Can you work these out from the model? Positions are in its coordinate system, mm. Face numbers are marked on the shaded views. Give positions to 0.01 mm unless a question says otherwise; leave off trailing zeros. Loops run counter-clockwise (first coordinate to the right, second up) from the corner with the lowest first, then second, coordinate; pieces in that order, holes last. Notation, with made-up numbers: M 69,10.5 L 100,10.5 A33 cw 100,42.5 Z; hole C 73,-23 d1. An arc over 180 degrees is marked long. One line per item, written item: value. Start each with the question number.
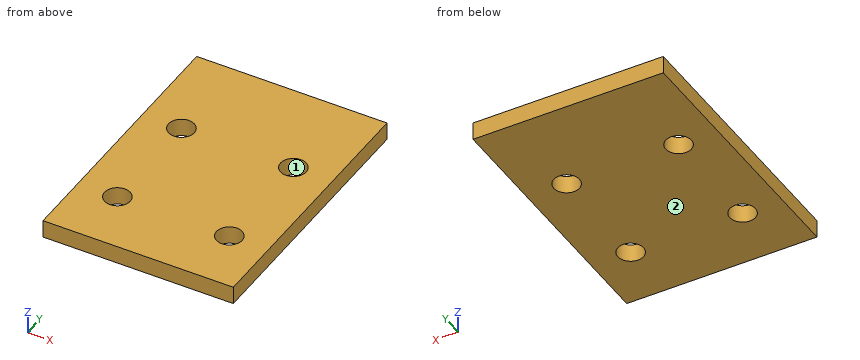
from build123d import *

# Parameters (mm, degrees)
SKETCH_1_W             = 170
SKETCH_1_H             = 240
SKETCH_1_R             = 11.5
SM_BASE_FLANGE_1_DEPTH = 16


# Sheet-metal steps are written as plain solids
with BuildPart() as part:
    # Sketch 1 → Базовая кромка1 (new body)
    with BuildSketch(Plane.XY):
        with Locations((85, -120)):
            Rectangle(SKETCH_1_W, SKETCH_1_H)
        with Locations((135, -185)):
            Circle(SKETCH_1_R, mode=Mode.SUBTRACT)
        with Locations((135, -85)):
            Circle(SKETCH_1_R, mode=Mode.SUBTRACT)
        with Locations(Location((35, -85, 0), (0, 0, 180))):
            Circle(SKETCH_1_R, mode=Mode.SUBTRACT)
        with Locations(Location((35, -185, 0), (0, 0, 180))):
            Circle(SKETCH_1_R, mode=Mode.SUBTRACT)
    extrude(amount=-SM_BASE_FLANGE_1_DEPTH)


solid = part.part
Q1. If we mould it in two halves opening along X, with no side actions, what happens to the marked faces 1 and 2? For each: released by +X, released by -X, zero draft, split by the parting line, or undercut.
Q2. For P1, Ø3, axis at x = 123.5, y = -139, coming from the +Z side, with a flat end and sliding along its axis, tell me the tip position at first contact or that it passes through.
Q3. If we section it at A-A, the plane y = -185: Write out the boundary of the cut face in (x, z), plus the area to 3 significant figures.
Q4. I need wall thicknesses on line 1 along Y through (x, z) = (135, -7); line 2 along Y through (x, z) = (42, -9.25); line 3 along X through (y, z) = (-88, -2.25). Which ranges of each line are inside material? Lowest first, please.
Q5. If we section it at C-C, the plane x = 141: Write out the boundary of the cut face in (y, z).
Q6. If we section it at B-B, the plane z = -13.5: Write out the boundary of the cut face in (x, y).
Response:
1. face 1: undercut
1. face 2: zero draft
2. P1: z = 0
3. outline: M 0,-16 L 23.5,-16 L 23.5,0 L 0,0 Z; M 46.5,-16 L 123.5,-16 L 123.5,0 L 46.5,0 Z; M 146.5,-16 L 170,-16 L 170,0 L 146.5,0 Z
3. area: 1,980 mm^2
4. line 1: -240 to -196.5, -173.5 to -96.5, -73.5 to 0
4. line 2: -240 to -194.12, -175.88 to -94.12, -75.88 to 0
4. line 3: 0 to 23.9, 46.1 to 123.9, 146.1 to 170
5. outline: M -240,-16 L -194.81,-16 L -194.81,0 L -240,0 Z; M -175.19,-16 L -94.81,-16 L -94.81,0 L -175.19,0 Z; M -75.19,-16 L 0,-16 L 0,0 L -75.19,0 Z
6. outline: M 0,-240 L 170,-240 L 170,0 L 0,0 Z; hole C 35,-185 d23; hole C 35,-85 d23; hole C 135,-185 d23; hole C 135,-85 d23
